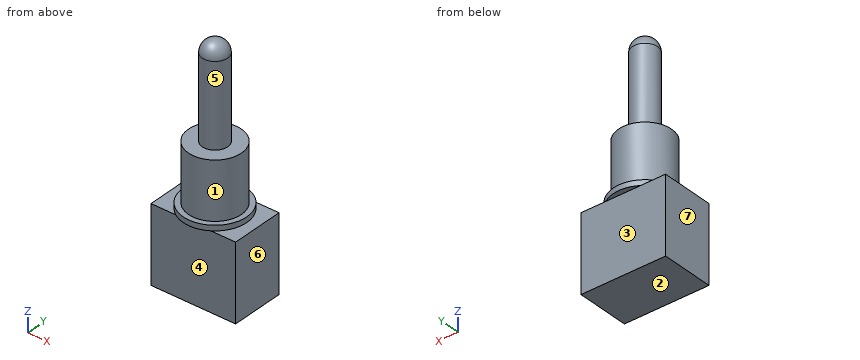
from build123d import *

# Parameters (mm, degrees)
F0_W     = 8
F0_H     = 5
F1_DEPTH = 7.2
F2_R     = 3
F3_DEPTH = 0.5
F4_R     = 2.5
F5_DEPTH = 5.4
F6_R     = 1.2
F7_DEPTH = 9
F8_R     = 1.2


with BuildPart() as f1:
    # F0 (on Top) → F1 (new body)
    with BuildSketch(Plane.XY):
        Rectangle(F0_W, F0_H)
    extrude(amount=F1_DEPTH)

    # F2 (on face) → F3 (join)
    with BuildSketch(Plane.XY.offset(7.2)):
        Circle(F2_R)
    extrude(amount=F3_DEPTH)

    # F4 (on face) → F5 (join)
    with BuildSketch(Plane.XY.offset(7.7)):
        Circle(F4_R)
    extrude(amount=F5_DEPTH)

    # F6 (on face) → F7 (join)
    with BuildSketch(Plane.XY.offset(13.1)):
        Circle(F6_R)
    extrude(amount=F7_DEPTH)

    # F8
    f8_edges = [f1.edges().sort_by_distance(p)[0] for p in [
        (-1.2, 0, 22.1),
    ]]
    fillet(f8_edges, radius=F8_R)


solid = f1.part
Read the model definition and answer for the solid it produces. Units are mm, in the model's axes. Face numbers are marked on the shaded views. A direction names the side the tool comes from. Give positions to 0.01 mm unless a question says otherwise; leave off trailing zeros. Write each loop counter-clockwise with the first axis right and the second up, starting at its lowest first coordinate (ties: lowest second). Pieces come first, ordered by that corner, then holes. Notation, with made-up numbers: (5, 6.5) - (46, 6.5) arc R14 cw to (46, 22.5) - close; hole circle Ø2 at (79.5, -24.75). An arc over 180 degrees is marked (long way). Use CSV: the item, a comma, the result in double quotes. Start each with the question number.
Item 1: The part is cut by section C-C, the plane z = 17.25. Give the vertices of the cut face in (x, y).
Item 2: The part is cut by section B-B, the plane x = 0. Give the vertices of the cut face in (y, z), and give its area (3 significant figures).
Item 3: Flat-ended cylindrical pins translate along their axes: P1, Ø2, axis at x = 3, y = -1, coming from the +Z side; P2, Ø2, axis at x = 1, z = 2, coming from the +Y side; P3, Ø2, axis at x = 0.5, z = 3.5, coming from the -Y side. Find the tip coordinate at first contact, or state that the pin passes through.
Item 4: The mould has two halves that part along X. Classify the marked faces 5, 6 and 7: pulls with the +X half, pulls with the -X half, needs draft (parallel to the pull), parting line crosses it, or undercut.
Item 5: For the marked faces 1, 2, 3 and 4, determine the directions among +Z, -Z, +X, -X, +Y, -Y from which every point of the face is accessible in a straight line to the end or side of a thin tool.
Item 6: Consider line 1 (Z direction, x = 0, y = -2.2); line 2 (Y direction, x = -2.75, z = 4.25); line 3 (Z direction, x = 2.25, y = 2.25). Determine where each line is inside the solid, lowest interval first.
Item 7: The part is cut by section A-A, the plane y = 0. Give the vertices of the cut face in (x, z), and give its area (3 significant figures).
Item 8: The part is cut by section D-D, the plane y = -1.45. Give the vertices of the cut face in (x, z), and give its area (3 significant figures).
Taken from the geometry:
1,outline,"circle Ø2.4 at (0, 0)"
2,outline,"(-3, 7.2) - (-2.5, 7.2) - (-2.5, 0) - (2.5, 0) - (2.5, 7.2) - (3, 7.2) - (3, 7.7) - (2.5, 7.7) - (2.5, 13.1) - (1.2, 13.1) - (1.2, 20.9) arc R1.2 ccw to (-1.2, 20.9) - (-1.2, 13.1) - (-2.5, 13.1) - (-2.5, 7.7) - (-3, 7.7) - close"
2,area,"87.0 mm2"
3,P1,"z = 13.1"
3,P2,"y = 2.5"
3,P3,"y = -2.5"
4,face 5,"parting line crosses it"
4,face 6,"pulls with the +X half"
4,face 7,"pulls with the -X half"
5,face 1,"+Z"
5,face 2,"-Z, +X, -X, +Y, -Y"
5,face 3,"-Z, +X, -X, +Y"
5,face 4,"-Z, +X, -X, -Y"
6,line 1,"0 to 13.1"
6,line 2,"-2.5 to 2.5"
6,line 3,"0 to 7.2"
7,outline,"(-4, 0) - (4, 0) - (4, 7.2) - (3, 7.2) - (3, 7.7) - (2.5, 7.7) - (2.5, 13.1) - (1.2, 13.1) - (1.2, 20.9) arc R1.2 ccw to (-1.2, 20.9) - (-1.2, 13.1) - (-2.5, 13.1) - (-2.5, 7.7) - (-3, 7.7) - (-3, 7.2) - (-4, 7.2) - close"
7,area,"109 mm2"
8,outline,"(-4, 0) - (4, 0) - (4, 7.2) - (2.63, 7.2) - (2.63, 7.7) - (2.04, 7.7) - (2.04, 13.1) - (-2.04, 13.1) - (-2.04, 7.7) - (-2.63, 7.7) - (-2.63, 7.2) - (-4, 7.2) - close"
8,area,"82.2 mm2"
